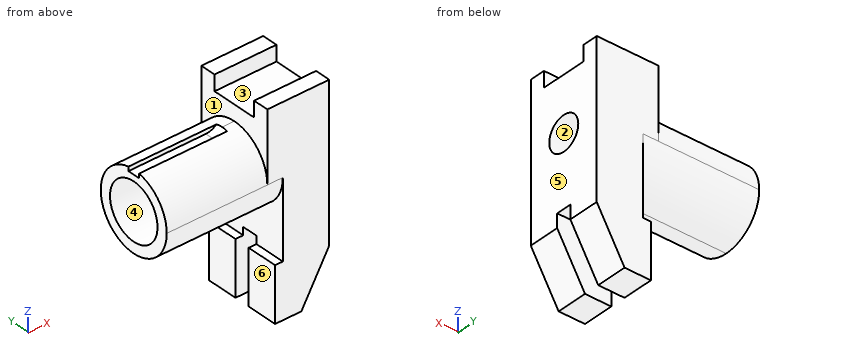
from build123d import *

# Parameters (mm, degrees)
EXTRUDE_1_DEPTH     = 25
CUT_EXTRUDE_1_REACH = 170.967
SKETCH_3_W          = 40
SKETCH_3_H          = 10
SKETCH_3_W_2        = 10
SKETCH_3_H_2        = 30
CUT_EXTRUDE_2_DEPTH = 75
CUT_EXTRUDE_3_DEPTH = 65
CUT_EXTRUDE_4_DEPTH = 4
SKETCH_8_R          = 18
CUT_EXTRUDE_5_DEPTH = 53
CUT_EXTRUDE_6_REACH = 144.597
SKETCH_9_R          = 11


with BuildPart() as part:
    # Эскиз1 → Бобышка-Вытянуть1 (new, symmetric)
    with BuildSketch(Plane(origin=(0, 0, 0), x_dir=(1, 0, 0), z_dir=(0, 1, 0))):
        Polygon((0, 0), (0, 98.823085464), (-18, 130), (-35, 130), (-35, 95), (-30, 95), (-30, 89.524477305), (-30, 70), (-105, 70), (-105, 20), (-40, 20), (-40, 0), align=None)
    extrude(amount=EXTRUDE_1_DEPTH, both=True)

    # Эскиз3 → Вырез-Вытянуть1 (cut, up to next)
    with BuildSketch(Plane(origin=(0, 0, 0), x_dir=(0, 0, -1), z_dir=(1, 0, 0)), mode=Mode.PRIVATE) as cut_extrude_1_sk1:
        with Locations((110, 0)):
            Rectangle(SKETCH_3_W, SKETCH_3_H)
    cut_extrude_1_tool1 = extrude(cut_extrude_1_sk1.sketch, amount=-CUT_EXTRUDE_1_REACH, mode=Mode.PRIVATE) & part.part
    # Эскиз3 → Вырез-Вытянуть1 (cut, up to next)
    with BuildSketch(Plane(origin=(0, 0, 0), x_dir=(0, 0, -1), z_dir=(1, 0, 0)), mode=Mode.PRIVATE) as cut_extrude_1_sk2:
        with Locations((5, 0)):
            Rectangle(SKETCH_3_W_2, SKETCH_3_H_2)
    cut_extrude_1_tool2 = extrude(cut_extrude_1_sk2.sketch, amount=-CUT_EXTRUDE_1_REACH, mode=Mode.PRIVATE) & part.part
    add(cut_extrude_1_tool1.solids().sort_by_distance((0, 0, -110))[0], mode=Mode.SUBTRACT)
    add(cut_extrude_1_tool2.solids().sort_by_distance((0, 0, -5))[0], mode=Mode.SUBTRACT)

    # Эскиз4 → Вырез-Вытянуть2 (cut)
    with BuildSketch(Plane.ZY.offset(105)):
        with BuildLine():
            Line((-70, -25), (-45, -25))
            ThreePointArc((-45, -25), (-62.677669515, -17.677669545), (-70, -4.2e-08))
            Line((-70, -4.2e-08), (-70, -25))
        make_face()
        with BuildLine():
            Line((-70, 25), (-70, -4.2e-08))
            ThreePointArc((-70, -4.2e-08), (-62.677669545, 17.677669515), (-45, 25))
            Line((-45, 25), (-70, 25))
        make_face()
    extrude(amount=-CUT_EXTRUDE_2_DEPTH, mode=Mode.SUBTRACT)

    # Эскиз6 → Вырез-Вытянуть3 (cut)
    with BuildSketch(Plane.ZY.offset(105)):
        with BuildLine():
            ThreePointArc((-20, 0), (-27.32233047, -17.67766953), (-45, -25))
            Line((-45, -25), (-20, -25))
            Line((-20, -25), (-20, 0))
        make_face()
        with BuildLine():
            ThreePointArc((-45, 25), (-27.32233047, 17.67766953), (-20, 0))
            Line((-20, 0), (-20, 25))
            Line((-20, 25), (-45, 25))
        make_face()
    extrude(amount=-CUT_EXTRUDE_3_DEPTH, mode=Mode.SUBTRACT)

    # Эскиз7 → Вырез-Вытянуть4 (cut, symmetric)
    with BuildSketch(Plane(origin=(0, 0, 0), x_dir=(1, 0, 0), z_dir=(0, 1, 0))):
        with BuildLine():
            Line((-105, 23), (-105, 20))
            Line((-105, 20), (-62.141428429, 20))
            ThreePointArc((-62.141428429, 20), (-58.872983346, 22.219544457), (-55, 23))
            Line((-55, 23), (-105, 23))
        make_face()
        with BuildLine():
            ThreePointArc((-55, 23), (-58.872983346, 22.219544457), (-62.141428429, 20))
            Line((-62.141428429, 20), (-55, 20))
            Line((-55, 20), (-55, 23))
        make_face()
        with BuildLine():
            ThreePointArc((-47.858571571, 20), (-51.127016654, 22.219544457), (-55, 23))
            Line((-55, 23), (-55, 20))
            Line((-55, 20), (-47.858571571, 20))
        make_face()
    extrude(amount=CUT_EXTRUDE_4_DEPTH, both=True, mode=Mode.SUBTRACT)

    # Эскиз8 → Вырез-Вытянуть5 (cut)
    with BuildSketch(Plane.ZY.offset(105)):
        with Locations((-45, 0)):
            Circle(SKETCH_8_R)
    extrude(amount=-CUT_EXTRUDE_5_DEPTH, mode=Mode.SUBTRACT)

    # Эскиз9 → Вырез-Вытянуть6 (cut, up to next)
    with BuildSketch(Plane.ZY.offset(52), mode=Mode.PRIVATE) as cut_extrude_6_sk1:
        with Locations((-45, 0)):
            Circle(SKETCH_9_R)
    cut_extrude_6_tool1 = extrude(cut_extrude_6_sk1.sketch, amount=-CUT_EXTRUDE_6_REACH, mode=Mode.PRIVATE) & part.part
    add(cut_extrude_6_tool1.solids().sort_by_distance((-52, 0, -45))[0], mode=Mode.SUBTRACT)


solid = part.part
Check sheet for the modelled part. Datum: model origin and axes. Units: mm. Face numbers are marked on the shaded views. A direction names the side the tool comes from. Round coordinates to 2 decimals unless told otherwise and drop trailing zeros. Loops run counter-clockwise (first coordinate to the right, second up) from the corner with the lowest first, then second, coordinate; pieces in that order, holes last. Notation, with made-up numbers: (44.5, 63) -> (101.5, 63) arc R26 cw to (101.5, 100) -> close; hole circle Ø9 at (80.25, -21). An arc over 180 degrees is marked (long way). Put each result on its own line as item: value. Start each with the question number.
1. Gauge pin test, flat ends, axial feed: pin 1 (1.5 mm diameter, centred on x = -44.5, y = -15.5, fed in from -Z); pin 2 (4 mm diameter, centred on y = 7.5, z = -89, fed in from -X); pin 3 (6 mm diameter, centred on y = 17.5, z = -113, fed in from -X); pin 4 (17.5 mm diameter, centred on y = 0, z = -45, fed in from -X). Record the tip position at first contact, or that the pin passes through.
2. Section check B-B (y = -9). Enter the section's corners in (x, z).
3. Access from +Z, -Z, +X, -X, +Y, -Y to the whole of each face (thin tool, end or side, straight path). Record for the marked faces 4, 5 and 6.
4. Section check A-A (x = -58). Enter the section's corners in (y, z).
5. Section check C-C (z = -117.5). Enter the section's corners in (x, y), plus the area to 3 significant figures.
6. Scan lines: probe 1 along Z at (x, y) = (-97, -1); probe 2 along Y at (x, z) = (-24.5, -101); probe 3 along Y at (x, z) = (-75.5, -45). Record each from-to range of solid material in increasing order.
7. Draft check along Z on the marked faces 1, 2 and 3. Enter one of: +Z half, -Z half, draft (parallel to the pull), parting line (faces both ways), or undercut.
8. Section check D-D (x = -21.5). Enter the section's corners in (y, z).
Findings:
1. pin 1: stops at z = -65.19
1. pin 2: stops at x = -30
1. pin 3: stops at x = -35
1. pin 4: passes through
2. outline: (-105, -68.32) -> (-30, -68.32) -> (-30, -95) -> (-35, -95) -> (-35, -130) -> (-18, -130) -> (0, -98.82) -> (0, -51.32) -> (-52, -51.32) -> (-52, -60.59) -> (-105, -60.59) -> close; (-105, -29.41) -> (-52, -29.41) -> (-52, -38.68) -> (0, -38.68) -> (0, -10) -> (-40, -10) -> (-40, -21.68) -> (-105, -21.68) -> close
3. face 4: -X
3. face 5: +Z, -Z, +X, +Y, -Y
3. face 6: -Z, -X, +Y, -Y
4. outline: (-4, -23) -> (-4, -20.32) arc R25 ccw (long way) to (4, -20.32) -> (4, -23) -> close; hole circle Ø36 at (0, -45)
5. outline: (-35, -25) -> (-10.78, -25) -> (-10.78, -5) -> (-35, -5) -> close; (-35, 5) -> (-10.78, 5) -> (-10.78, 25) -> (-35, 25) -> close
5. area: 969 mm^2
6. probe 1: z = -69.98 to -62.97, -27.03 to -23
6. probe 2: y = -25 to -5, 5 to 25
6. probe 3: y = -25 to -18, 18 to 25
7. face 1: draft
7. face 2: undercut
7. face 3: +Z half
8. outline: (-25, -130) -> (-5, -130) -> (-5, -90) -> (5, -90) -> (5, -130) -> (25, -130) -> (25, 0) -> (15, 0) -> (15, -10) -> (-15, -10) -> (-15, 0) -> (-25, 0) -> close; hole circle Ø22 at (0, -45)
